```python
from build123d import *

# Parameters (mm, degrees)
F0_W          = 127
F0_H          = 127
F1_DEPTH      = 25.4
F1_DEPTH_BACK = 25.4
F2_W          = 114.3
F2_H          = 114.3
F3_DEPTH      = 44.45
F4_R          = 12.7


with BuildPart() as f1:
    # F0 (on Front) → F1 (new body, two sides)
    with BuildSketch(Plane.XZ) as f1_sk:
        with Locations((-4.264493, -4.37899)):
            Rectangle(F0_W, F0_H)
    extrude(amount=F1_DEPTH)
    extrude(f1_sk.sketch, amount=-F1_DEPTH_BACK)

    # F2 (on face) → F3 (cut)
    with BuildSketch(Plane.XZ.offset(25.4)):
        with Locations((-4.264493, -4.37899)):
            Rectangle(F2_W, F2_H)
    extrude(amount=-F3_DEPTH, mode=Mode.SUBTRACT)

    # F4
    f4_edges = [f1.edges().sort_by_distance(p)[0] for p in [
        (-61.414493, -3.175, -61.52899),
        (52.885507, -3.175, -61.52899),
        (52.885507, -3.175, 52.77101),
        (-61.414493, -3.175, 52.77101),
    ]]
    fillet(f4_edges, radius=F4_R)


solid = f1.part
```
Geometry: final body of the model. Coordinates: model frame, mm. A direction names the side the tool comes from. Give positions to 0.01 mm unless a question says otherwise; leave off trailing zeros. Order: outer loops, then holes, each group sorted by start corner. A loop starts at its lowest first (then second) coordinate and runs counter-clockwise, first axis right, second up. Notation, with made-up numbers: M 30.25,62.25 L 42.25,62.25 A15 cw 42.25,90.25 Z; hole C 78,59.25 d6. An arc over 180 degrees is marked long. Answer as CSV lines item,"result". Start each with the question number.
1) Set-up query: faces 4 (the flat face through (-5, 19.05, -4)), 5 (the flat face through (-67.764, 0, -5)). Return all of +Z, -Z, +X, -X, +Y, -Y with unobstructed straight access to the full face (end or side cutting, diameter ignored); none if empty.
2) Mould query, pull axis Z, two halves, no side actions, for faces 1 (the flat face through (-9, -25.4, -65)), 2 (the flat face through (-5, 0, 59.121)), 3 (the flat face through (52.886, -3, -5)). Classes: +Z half, -Z half, draft (parallel to the pull), parting line (faces both ways), or undercut.
3) Cut plane A-A (x = -40.5). Output: boundary loops of the cut face in (y, z), then the cut area to 3 significant figures.
4) Cut plane B-B (y = -14). Output: boundary loops of the cut face in (x, z), then the cut area to 3 significant figures.
5) Line query: line 1 (Z direction, x = 8.5, y = 18.5); line 2 (X direction, y = -10, z = -45); line 3 (Y direction, x = 5, z = -22.5). Output: solid intervals per line, ascending. Write a range as from..to.
6) Cut plane C-C (z = 28). Output: boundary loops of the cut face in (x, y).
7) First-contact query: P1, Ø8, axis at x = 41, z = -11.5, coming from the -Y side. Flat tip, straight axial feed; report the tip coordinate or a pass-through.
Findings below:
1,face 4,"-Y"
1,face 5,"+Z, -Z, -X, +Y, -Y"
2,face 1,"draft"
2,face 2,"+Z half"
2,face 3,"undercut"
3,outline,"M -25.4,-67.88 L 25.4,-67.88 L 25.4,59.12 L -25.4,59.12 L -25.4,52.77 L 19.05,52.77 L 19.05,-61.53 L -25.4,-61.53 Z"
3,area,"1,370 mm²"
4,outline,"M -67.76,-67.88 L 59.24,-67.88 L 59.24,59.12 L -67.76,59.12 Z; hole M -61.41,-48.83 A12.7 ccw -48.71,-61.53 L 40.19,-61.53 A12.7 ccw 52.89,-48.83 L 52.89,40.07 A12.7 ccw 40.19,52.77 L -48.71,52.77 A12.7 ccw -61.41,40.07 Z"
4,area,"3,200 mm²"
5,line 1,"z = -67.88..-61.53, 52.77..59.12"
5,line 2,"x = -67.76..-61.41, 52.89..59.24"
5,line 3,"y = 19.05..25.4"
6,outline,"M -67.76,-25.4 L -61.41,-25.4 L -61.41,19.05 L 52.89,19.05 L 52.89,-25.4 L 59.24,-25.4 L 59.24,25.4 L -67.76,25.4 Z"
7,P1,"stops at y = 19.05"
